The listing builds one solid part. Answer for the finished solid, in the listing's coordinates (mm). Give positions to 0.01 mm unless a question says otherwise; leave off trailing zeros. Write each loop counter-clockwise with the first axis right and the second up, starting at its lowest first coordinate (ties: lowest second). Pieces come first, ordered by that corner, then holes. Notation, with made-up numbers: M -33.5,19 L -17.5,19 A11 ccw -17.5,32 Z; hole C -20.75,54 d4. An arc over 180 degrees is marked long. Return JSON: item names as keys, results as strings.
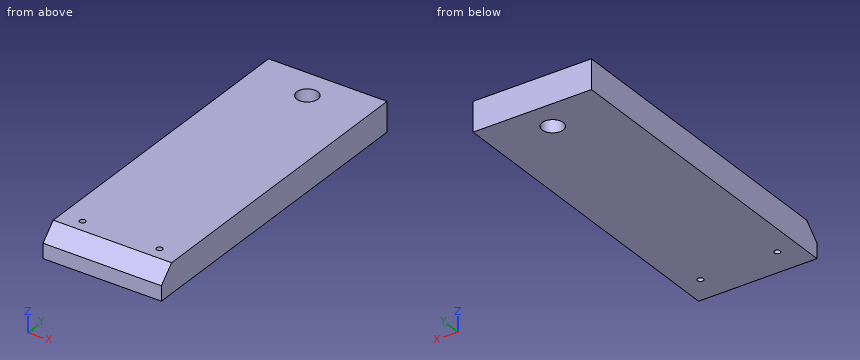
from build123d import *

# Parameters (mm, degrees)
SKETCH1_W           = 25.4
SKETCH1_H           = 69.85
BOSS_EXTRUDE1_DEPTH = 6.35
SKETCH2_R           = 2.25
SKETCH2_R_2         = 0.625
CUT_EXTRUDE1_DEPTH  = 6.35
CHAMFER1_SIZE       = 3.175


with BuildPart() as part:
    # Sketch1 → Boss-Extrude1 (new body)
    with BuildSketch(Plane.XY):
        with Locations((12.7, 34.925)):
            Rectangle(SKETCH1_W, SKETCH1_H)
    extrude(amount=BOSS_EXTRUDE1_DEPTH)

    # Sketch2 → Cut-Extrude1 (cut)
    with BuildSketch(Plane.XY.offset(6.35)):
        with Locations((12.7, 63.5)):
            Circle(SKETCH2_R)
        with Locations((4.445, 5.842)):
            Circle(SKETCH2_R_2)
        with Locations((20.955, 5.842)):
            Circle(SKETCH2_R_2)
    extrude(amount=-CUT_EXTRUDE1_DEPTH, mode=Mode.SUBTRACT)

    # Chamfer1
    chamfer1_edges = [part.edges().sort_by_distance(p)[0] for p in [
        (12.7, 0, 6.35),
    ]]
    chamfer(chamfer1_edges, length=CHAMFER1_SIZE)


solid = part.part
Item 1: A cutting plane is placed at A-A, the plane x = 12.7. Write down the section's boundary in (y, z) (3 decimals).
Geometry results:
{"outline": "M 0,0 L 61.25,0 L 61.25,6.35 L 3.175,6.35 L 0,3.175 Z; M 65.75,0 L 69.85,0 L 69.85,6.35 L 65.75,6.35 Z"}
Item 2: Given pin 1 Ø4 at (x, y) = (10.5, 46) entering from -Z, flat-ended and moving along its own axis, determine where the tip first touches the part or whether it passes through.
Geometry results:
{"pin 1": "stops at z = 0"}
Item 3: A cutting plane is placed at B-B, the plane y = 63.5. Write down the section's boundary in (x, z).
Geometry results:
{"outline": "M 0,0 L 10.45,0 L 10.45,6.35 L 0,6.35 Z; M 14.95,0 L 25.4,0 L 25.4,6.35 L 14.95,6.35 Z"}
Item 4: A cutting plane is placed at C-C, the plane z = 5.5. Write down the section's boundary in (x, y) (3 decimals), plus the area to 3 significant figures.
Geometry results:
{"outline": "M 0,2.325 L 25.4,2.325 L 25.4,69.85 L 0,69.85 Z; hole C 4.445,5.842 d1.25; hole C 12.7,63.5 d4.5; hole C 20.955,5.842 d1.25", "area": "1,700 mm2"}
Item 5: Find the intervals of material crossed by line 1 (Y direction, x = 12.7, z = 2.75); line 2 (Y direction, x = 4.25, z = 3.75) (3 decimals); line 3 (X direction, y = 62, z = 3.75), in increasing order.
Geometry results:
{"line 1": "y = 0 to 61.25, 65.75 to 69.85", "line 2": "y = 0.575 to 5.248, 6.436 to 69.85", "line 3": "x = 0 to 11.02, 14.38 to 25.4"}
